from build123d import *

# Parameters (mm, degrees)
SKETCH1_R           = 4.572
BOSS_EXTRUDE1_DEPTH = 5.08
SKETCH2_R           = 3.1115
CUT_EXTRUDE1_DEPTH  = 3.81
SKETCH3_R           = 4.064
SKETCH3_R_2         = 2.794
EXTRUDE_THIN1_DEPTH = 3.81


with BuildPart() as part:
    # Sketch1 → Boss-Extrude1 (new body)
    with BuildSketch(Plane(origin=(0, 0, 0), x_dir=(1, 0, 0), z_dir=(0, 1, 0))):
        with Locations(Location((0, 0, 0), (0, 0, 270))):
            Circle(SKETCH1_R)
    extrude(amount=BOSS_EXTRUDE1_DEPTH)

    # Sketch2 → Cut-Extrude1 (cut)
    with BuildSketch(Plane(origin=(0, 5.08, 0), x_dir=(1, 0, 0), z_dir=(0, 1, 0))):
        with Locations(Location((0, 0, 0), (0, 0, 270))):
            Circle(SKETCH2_R)
    extrude(amount=-CUT_EXTRUDE1_DEPTH, mode=Mode.SUBTRACT)

    # Sketch3 → Extrude-Thin1 (add)
    with BuildSketch(Plane(origin=(0, 0, 0), x_dir=(-1, 0, 0), z_dir=(0, -1, 0))):
        Circle(SKETCH3_R)
        Circle(SKETCH3_R_2, mode=Mode.SUBTRACT)
    extrude(amount=EXTRUDE_THIN1_DEPTH)


solid = part.part
Check sheet for the modelled part. Datum: model origin and axes. Units: mm. A direction names the side the tool comes from. Round coordinates to 2 decimals unless told otherwise and drop trailing zeros. Loops run counter-clockwise (first coordinate to the right, second up) from the corner with the lowest first, then second, coordinate; pieces in that order, holes last. Notation, with made-up numbers: (63.5, 74) -> (114.5, 74) arc R20 ccw to (114.5, 110) -> close; hole circle Ø4 at (21, 56). An arc over 180 degrees is marked (long way). Put each result on its own line as item: value. Start each with the question number.
1. Draft check along X on faces 3 (the face through (-4.056, 2.504, 2.11)), 4 (the face through (0, 0, 0)), 5 (the face through (1, -3.81, 3)). Enter one of: +X half, -X half, draft (parallel to the pull), parting line (faces both ways), or undercut.
2. Gauge pin test, flat ends, axial feed: pin 1 (1.9 mm diameter, centred on x = 0.5, z = 0.5, fed in from +Y); pin 2 (1 mm diameter, centred on x = 1, y = 2.5, fed in from +Z); pin 3 (2 mm diameter, centred on y = 1, z = -3, fed in from +X). Record the tip position at first contact, or that the pin passes through.
3. Access from +Z, -Z, +X, -X, +Y, -Y to the whole of each face (thin tool, end or side, straight path). Record for faces 1 (the face through (-3.04, 3.2, -0.67)), 2 (the face through (0.881, -1.878, 3.967)).
4. Section check A-A (x = 0). Enter the section's corners in (y, z).
5. Scan lines: probe 1 along Z at (x, y) = (0, -2.1); probe 2 along X at (y, z) = (3.7, 0). Record each from-to range of solid material in increasing order.
6. Section check B-B (z = 0). Enter the section's corners in (x, y).
7. Section check D-D (z = -3.5). Enter the section's corners in (x, y), plus the area to 3 significant figures.
8. Section check C-C (y = 0.5). Enter the section's corners in (x, z), plus the area to 3 significant figures.
Findings:
1. face 3: parting line
1. face 4: undercut
1. face 5: draft
2. pin 1: stops at y = 1.27
2. pin 2: stops at z = 4.54
2. pin 3: stops at x = 4.11
3. face 1: +Y
3. face 2: -Y
4. outline: (-3.81, -4.06) -> (0, -4.06) -> (0, -4.57) -> (5.08, -4.57) -> (5.08, -3.11) -> (1.27, -3.11) -> (1.27, 3.11) -> (5.08, 3.11) -> (5.08, 4.57) -> (0, 4.57) -> (0, 4.06) -> (-3.81, 4.06) -> (-3.81, 2.79) -> (0, 2.79) -> (0, -2.79) -> (-3.81, -2.79) -> close
5. probe 1: z = -4.06 to -2.79, 2.79 to 4.06
5. probe 2: x = -4.57 to -3.11, 3.11 to 4.57
6. outline: (-4.57, 0) -> (-4.06, 0) -> (-4.06, -3.81) -> (-2.79, -3.81) -> (-2.79, 0) -> (2.79, 0) -> (2.79, -3.81) -> (4.06, -3.81) -> (4.06, 0) -> (4.57, 0) -> (4.57, 5.08) -> (3.11, 5.08) -> (3.11, 1.27) -> (-3.11, 1.27) -> (-3.11, 5.08) -> (-4.57, 5.08) -> close
7. outline: (-2.94, 0) -> (-2.07, 0) -> (-2.07, -3.81) -> (2.07, -3.81) -> (2.07, 0) -> (2.94, 0) -> (2.94, 5.08) -> (-2.94, 5.08) -> close
7. area: 45.6 mm^2
8. outline: circle Ø9.14 at (0, 0)
8. area: 65.7 mm^2
